The listing builds one solid part. Answer for the finished solid, in the listing's coordinates (mm). Face numbers are marked on the shaded views. Round coordinates to 2 decimals unless told otherwise and drop trailing zeros. Put each result on its own line as item: value. Start each with the question number.
```python
from build123d import *

# Parameters (mm, degrees)
ESBO_O1_W                 = 6.5
ESBO_O1_H                 = 3.56
EXTRUS_O1_DEPTH           = 0.9
EXTRUS_O1_TAPER           = 6
EXTRUS_O1_OTHER_WAY_DEPTH = 0.7
EXTRUS_O1_OTHER_WAY_TAPER = 6
ESBO_O3_W                 = 0.74
ESBO_O3_H                 = 0.3
PADR_O_LINEAR1_COUNT      = 2
PADR_O_LINEAR1_PITCH      = 2.3
PADR_O_LINEAR1_COL_COUNT  = 2
PADR_O_LINEAR1_COL_PITCH  = 2.3
ESBO_O5_W                 = 4
ESBO_O5_H                 = 0.3


with BuildPart() as part:
    # Esboço1 → Extrusão1 (new body)
    with BuildSketch(Plane(origin=(0, 0, 0), x_dir=(1, 0, 0), z_dir=(0, 1, 0))):
        Rectangle(ESBO_O1_W, ESBO_O1_H)
    extrude(amount=EXTRUS_O1_DEPTH, taper=EXTRUS_O1_TAPER)

    # Esboço1 → Extrusão1 other way (add)
    with BuildSketch(Plane(origin=(0, 0, 0), x_dir=(1, 0, 0), z_dir=(0, 1, 0))):
        Rectangle(ESBO_O1_W, ESBO_O1_H)
    extrude(amount=-EXTRUS_O1_OTHER_WAY_DEPTH, taper=EXTRUS_O1_OTHER_WAY_TAPER)

    # Varredura1: sweep along a path in Esboço2
    with BuildLine(Plane(origin=(0, 0, 0), x_dir=(0, 0, -1), z_dir=(1, 0, 0))) as varredura1_path:
        Line((-1.771086264, -0.084808537), (-2.138904869, -0.084808537))
        ThreePointArc((-2.138904869, -0.084808537), (-2.349489276, -0.131317404), (-2.520897515, -0.262191707))
        Line((-2.520897515, -0.262191707), (-2.752531862, -0.536457055))
        ThreePointArc((-2.752531862, -0.536457055), (-2.88725344, -0.648417053), (-3.052325014, -0.707037188))
        Line((-3.052325014, -0.707037188), (-3.471086264, -0.776830729))
    # Esboço3 → Varredura1 (sweep)
    with BuildSketch(Plane(origin=(0, -0.185041405, 1.760551365), x_dir=(1, 0, 0), z_dir=(0, -0.104528463, 0.994521895))):
        with Locations((0, 0.023347308)):
            Rectangle(ESBO_O3_W, ESBO_O3_H)
    varredura1 = sweep(path=varredura1_path.line)

    # Padrão linear1: Varredura1 ×2
    with Locations(*[(i * PADR_O_LINEAR1_PITCH, 0, 0) for i in range(1, PADR_O_LINEAR1_COUNT)]):
        add(varredura1)

    # Padrão linear1 col: Varredura1 ×2
    with Locations(*[(-i * PADR_O_LINEAR1_COL_PITCH, 0, 0) for i in range(1, PADR_O_LINEAR1_COL_COUNT)]):
        add(varredura1)

    # Varredura2: sweep along a path in Esboço4
    with BuildLine(Plane(origin=(0, 0, 0), x_dir=(0, 0, -1), z_dir=(1, 0, 0))) as varredura2_path:
        Line((1.770334988, -0.091956448), (2.13866613, -0.091956448))
        ThreePointArc((2.13866613, -0.091956448), (2.34886791, -0.138287834), (2.52011393, -0.2686956))
        Line((2.52011393, -0.2686956), (2.751853347, -0.542148112))
        ThreePointArc((2.751853347, -0.542148112), (2.886396765, -0.653672528), (3.051101653, -0.712084226))
        Line((3.051101653, -0.712084226), (3.470334988, -0.781956448))
    # Esboço5 → Varredura2 (sweep)
    with BuildSketch(Plane(origin=(0, -0.185041405, -1.760551365), x_dir=(-1, 0, 0), z_dir=(0, -0.104528463, -0.994521895))):
        with Locations((0, 0.014790466)):
            Rectangle(ESBO_O5_W, ESBO_O5_H)
    sweep(path=varredura2_path.line)


solid = part.part
```
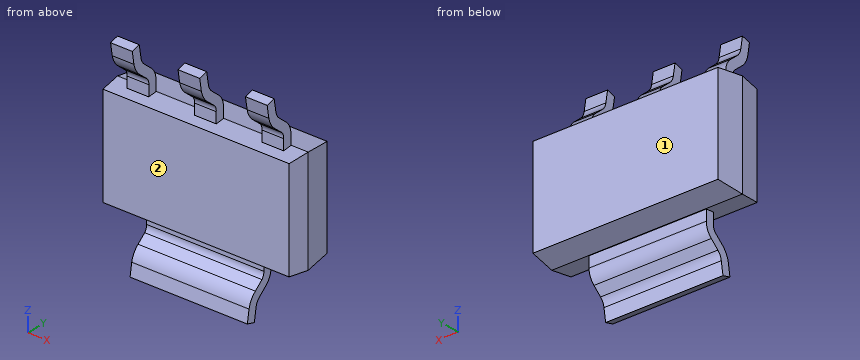
Item 1: Determine the mould class of the marked faces 1 and 2 for opening direction Z: released by +Z, released by -Z, zero draft, split by the parting line, or undercut.
Item 2: Flat-ended cylindrical pins translate along their axes: pin 1 (0.5 mm diameter, centred on y = -0.5, z = 3, fed in from -X); pin 2 (0.8 mm diameter, centred on y = -0.5, z = -2.5, fed in from -X); pin 3 (1.5 mm diameter, centred on x = -1, z = -2, fed in from +Y); pin 4 (1.1 mm diameter, centred on y = -0.5, z = -2.5, fed in from +X). Find the tip coordinate at first contact, or state that the pin passes through.
Item 3: Consider line 1 along X through (y, z) = (-0.35, 2.5); line 2 along X through (y, z) = (0.7, 0); line 3 along Z through (x, y) = (2.75, 0.7). Determine where each line is inside the solid, lowest interval first. Write a range as [from, to].
Output values:
1. face 1: zero draft
1. face 2: undercut
2. pin 1: stops at x = -2.67
2. pin 2: stops at x = -2
2. pin 3: stops at y = 0.9
2. pin 4: stops at x = 2
3. line 1: x = [-2.67, -1.93], [-0.37, 0.37], [1.93, 2.67]
3. line 2: x = [-3.18, 3.18]
3. line 3: z = [-1.71, 1.71]
